from build123d import *

# Parameters (mm, degrees)
SKETCH1_W           = 105
SKETCH1_H           = 22.5
BOSS_EXTRUDE1_DEPTH = 2.5
SKETCH2_W           = 105
SKETCH2_H           = 2.5
BOSS_EXTRUDE2_DEPTH = 20
CUT_EXTRUDE1_DEPTH  = 59.215655111
FILLET1_R           = 1


with BuildPart() as part:
    # Sketch1 → Boss-Extrude1 (new body)
    with BuildSketch(Plane(origin=(0, 0, 0), x_dir=(1, 0, 0), z_dir=(0, 1, 0))):
        Rectangle(SKETCH1_W, SKETCH1_H)
    extrude(amount=BOSS_EXTRUDE1_DEPTH)

    # Sketch2 → Boss-Extrude2 (add)
    with BuildSketch(Plane(origin=(0, 2.5, 0), x_dir=(1, 0, 0), z_dir=(0, 1, 0))):
        with Locations((0, 10)):
            Rectangle(SKETCH2_W, SKETCH2_H)
    extrude(amount=BOSS_EXTRUDE2_DEPTH)

    # Sketch3 → Cut-Extrude1 (cut, through all)
    with BuildSketch(Plane(origin=(0, 0, 0), x_dir=(-1, 0, 0), z_dir=(0, -1, 0))):
        Polygon((52.5, -11.25), (52.5, 11.25), (30, -11.25), align=None)
    extrude(amount=-CUT_EXTRUDE1_DEPTH, mode=Mode.SUBTRACT)

    # Fillet1
    fillet1_edges = [part.edges().sort_by_distance(p)[0] for p in [
        (0, 22.5, -11.25),
        (1.25, 22.5, -8.75),
        (1.25, 2.5, -8.75),
        (11.25, 0, 11.25),
        (11.25, 2.5, 11.25),
        (0, 0, -11.25),
    ]]
    fillet(fillet1_edges, radius=FILLET1_R)


solid = part.part
Model file for the job. Use its own axes, mm. A direction names the side the tool comes from. Give positions to 0.01 mm unless a question says otherwise; leave off trailing zeros. Write each loop counter-clockwise with the first axis right and the second up, starting at its lowest first coordinate (ties: lowest second). Pieces come first, ordered by that corner, then holes. Notation, with made-up numbers: M 59.25,-25.5 L 118.25,-25.5 A27 cw 118.25,-6.5 Z; hole C 53,-27 d4. An arc over 180 degrees is marked long. One line per item, written item: value. Start each with the question number.
Q1. Saw through at A-A, the plane x = 4.5. Write the cut outline in (y, z), plus the area to 3 significant figures.
Q2. Drop flat-ended pins along their axis: pin 1 Ø4 at (x, z) = (-34, -5.5) entering from +Y; pin 2 Ø5 at (y, z) = (18.5, -5) entering from -X. Give the stop position or say it passes through.
Q3. Saw through at B-B, the plane z = 2.25. Write the cut outline in (x, y).
Q4. Saw through at D-D, the plane x = -40. Write the cut outline in (y, z).
Q5. 3-axis set-ups, long thin cutter, end or side, ignore diameter. For faces 1 (the flat face through (1, 12, -8.75)), 2 (the flat face through (-46.3, 2.03, -5.05)): which of +Z, -Z, +X, -X, +Y, -Y reach the whole face in a straight line?
Q6. Saw through at C-C, the plane y = 9. Write the cut outline in (x, z), plus the area to 3 significant figures.
Q7. Probe probe 1 along Z at (x, y) = (11.5, 14.25); probe 2 along Y at (x, z) = (-14, 9.75); probe 3 along X at (y, z) = (20, -9.25). List the from-to ranges inside material, lowest first. Write a range as [from, to].
Output values:
1. outline: M 0,-10.25 A1 ccw 1,-11.25 L 21.5,-11.25 A1 ccw 22.5,-10.25 L 22.5,-9.75 A1 ccw 21.5,-8.75 L 3.5,-8.75 A1 cw 2.5,-7.75 L 2.5,10.25 A1 ccw 1.5,11.25 L 1,11.25 A1 ccw 0,10.25 Z
1. area: 105 mm²
2. pin 1: stops at y = 2.5
2. pin 2: passes through
3. outline: M -39,0 L 52.5,0 L 52.5,2.5 L -39,2.5 Z
4. outline: M 0,-10.25 A1 ccw 1,-11.25 L 21.5,-11.25 A1 ccw 22.5,-10.25 L 22.5,-9.75 A1 ccw 21.5,-8.75 L 3.5,-8.75 A1 cw 2.5,-7.75 L 2.5,1.25 L 0,1.25 Z
5. face 1: +Z, +X, -X, +Y
5. face 2: +Z, -X, +Y, -Y
6. outline: M -52.5,-11.25 L 52.5,-11.25 L 52.5,-8.75 L -50,-8.75 Z
6. area: 259 mm²
7. probe 1: z = [-11.25, -8.75]
7. probe 2: y = [0, 2.5]
7. probe 3: x = [-50.5, 52.5]
